```python
from build123d import *
from build123d.topology import SkipClean

# Parameters (mm, degrees)
SKETCH1_R           = 10
SKETCH1_R_2         = 5
BOSS_EXTRUDE1_DEPTH = 5
BOSS_EXTRUDE2_START = 6
SKETCH3_R           = 17.5
SKETCH3_R_2         = 5
BOSS_EXTRUDE2_DEPTH = 6
CUT_EXTRUDE1_DEPTH  = 3
SKETCH5_W           = 2.5
SKETCH5_H           = 2.5
CUT_EXTRUDE2_DEPTH  = 10


with BuildPart() as part:
    # Sketch1 → Boss-Extrude1 (new, symmetric)
    with BuildSketch(Plane.XY):
        Circle(SKETCH1_R)
        Circle(SKETCH1_R_2, mode=Mode.SUBTRACT)
    extrude(amount=BOSS_EXTRUDE1_DEPTH, both=True)

    # Sketch3 → Boss-Extrude2 (add)
    with SkipClean():  # the faces are left unmerged after this step: merging them gives an invalid solid
        with BuildSketch(Plane(origin=(0, 0, -5), x_dir=(-1, 0, 0), z_dir=(0, 0, -1)).offset(BOSS_EXTRUDE2_START)):
            Circle(SKETCH3_R)
            Circle(SKETCH3_R_2, mode=Mode.SUBTRACT)
        extrude(amount=-BOSS_EXTRUDE2_DEPTH)

    # Sketch4 → Cut-Extrude1 (cut)
    with SkipClean():  # the faces are left unmerged after this step: merging them gives an invalid solid
        with BuildSketch(Plane(origin=(0, 0, -11), x_dir=(-1, 0, 0), z_dir=(0, 0, -1))):
            with BuildLine():
                Line((-16.770509831, -5), (16.770509831, -5))
                ThreePointArc((16.770509831, -5), (17.5, 0), (16.770509831, 5))
                Line((16.770509831, 5), (-16.770509831, 5))
                ThreePointArc((-16.770509831, 5), (-17.5, 0), (-16.770509831, -5))
            make_face()
        extrude(amount=-CUT_EXTRUDE1_DEPTH, mode=Mode.SUBTRACT)

    # Sketch5 → Cut-Extrude2 (cut)
    with SkipClean():  # the faces are left unmerged after this step: merging them gives an invalid solid
        with BuildSketch(Plane.XY.offset(5)):
            with Locations((5, 0)):
                Rectangle(SKETCH5_W, SKETCH5_H)
        extrude(amount=-CUT_EXTRUDE2_DEPTH, mode=Mode.SUBTRACT)


solid = part.part
```
Input: part model. Units: mm. Frame: model coordinates. A direction names the side the tool comes from. Give positions to 0.01 mm unless a question says otherwise; leave off trailing zeros. Write each loop counter-clockwise with the first axis right and the second up, starting at its lowest first coordinate (ties: lowest second). Pieces come first, ordered by that corner, then holes. Notation, with made-up numbers: (3, 10) - (31, 10) arc R4 ccw to (31, 16) - close; hole circle Ø5 at (67.25, 14). An arc over 180 degrees is marked (long way). Write item = value, one per line. Start each with the question number.
1) Pin query (flat end, axial travel): pin 1 (2 mm diameter, centred on x = -1.5, y = -2, fed in from -Z); pin 2 (3.5 mm diameter, centred on x = -4.5, z = -10, fed in from +Y); pin 3 (1.2 mm diameter, centred on y = 0, z = -2.5, fed in from -X); pin 4 (1.5 mm diameter, centred on x = 5, z = -10, fed in from -Y). Return the tip coordinate at first contact, or that it passes through.
2) Cut plane B-B (x = -3). Return loops of the section in (y, z), and give its area (3 significant figures).
3) Material intervals for L1, parallel to Y at x = 0, z = -3.25; L2, parallel to Z at x = 0, y = -13; L3, parallel to X at y = -1, z = -2.5, sorted ascending. Write a range as [from, to].
4) Draft query along Y for faces 4 (the face through (0, 5, -10)), 5 (the face through (-16.69, 5.26, -8.04)), 6 (the face through (0, 10, -11)). Return one class per face: pulls with the +Y half, pulls with the -Y half, needs draft (parallel to the pull), parting line crosses it, or undercut.
5) Cut plane D-D (x = -14.5). Return loops of the section in (y, z), and give its area (3 significant figures).
6) Reachability of faces 1 (the face through (11, 0, -8)), 2 (the face through (0, -10, -11)), 3 (the face through (6.25, 0, 0)) from +Z, -Z, +X, -X, +Y, -Y: full face, straight path, thin tool, end or side. Return the list, or none.
7) Cut plane A-A (y = 0). Return loops of the section in (x, z), and give its area (4 significant figures).
8) Cut plane C-C (z = 1.75). Return loops of the section in (x, y).
Answers follow:
q1.pin_1 = through
q1.pin_2 = 17.28
q1.pin_3 = -10
q1.pin_4 = -16.98
q2.outline = (-17.24, -11) - (-5, -11) - (-5, -8) - (-4, -8) - (-4, 5) - (-9.54, 5) - (-9.54, -5) - (-17.24, -5) - close; (4, -8) - (5, -8) - (5, -11) - (17.24, -11) - (17.24, -5) - (9.54, -5) - (9.54, 5) - (4, 5) - close
q2.area = 264 mm^2
q3.L1 = [-10, -5], [5, 10]
q3.L2 = [-11, -5]
q3.L3 = [-9.95, -4.9], [6.25, 9.95]
q4.face_4 = undercut
q4.face_5 = parting line crosses it
q4.face_6 = needs draft
q5.outline = (-9.8, -11) - (-5, -11) - (-5, -8) - (5, -8) - (5, -11) - (9.8, -11) - (9.8, -5) - (-9.8, -5) - close
q5.area = 87.6 mm^2
q6.face_1 = -Z, +X, -X
q6.face_2 = -Z, +X, -X, +Y, -Y
q6.face_3 = +Z
q7.outline = (-17.5, -8) - (-5, -8) - (-5, 5) - (-10, 5) - (-10, -5) - (-17.5, -5) - close; (5, -8) - (17.5, -8) - (17.5, -5) - (10, -5) - (10, 5) - (6.25, 5) - (6.25, -5) - (5, -5) - close
q7.area = 162.5 mm^2
q8.outline = circle Ø20 at (0, 0); hole (4.84, -1.25) - (6.25, -1.25) - (6.25, 1.25) - (4.84, 1.25) arc R5 ccw (long way) to start
